Geometry check sheet. Reference: drawing and pictorial views, mm from the part's lowest x, y, z. A direction names the side the tool comes from. Round coordinates to 2 decimals unless told otherwise and drop trailing zeros. Write each loop counter-clockwise with the first axis right and the second up, starting at its lowest first coordinate (ties: lowest second). Pieces come first, ordered by that corner, then holes. Notation, with made-up numbers: (-11.5, 10.5) - (-4.5, 10.5) arc R34 cw to (-4.5, 46.5) - close; hole circle Ø5 at (2, -13.5). An arc over 180 degrees is marked (long way). Return JSON: item names as keys, results as strings.
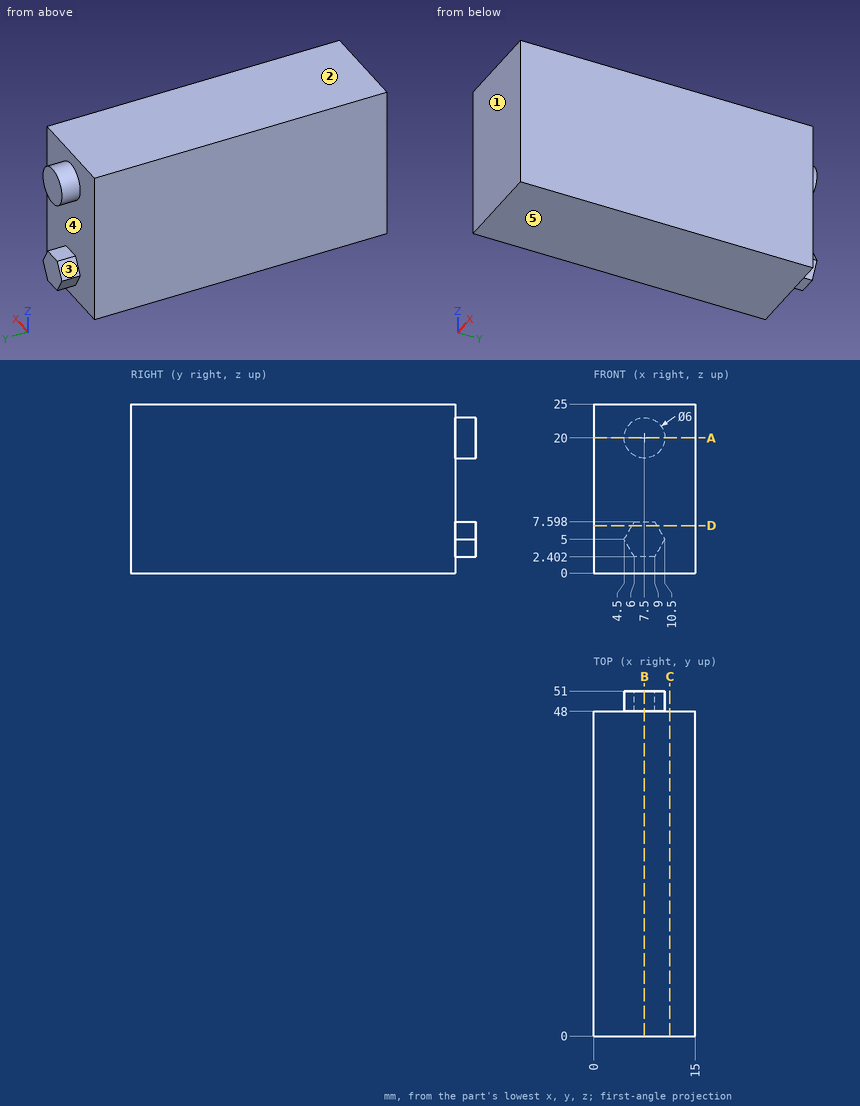
(1) Section check B-B, the plane x = 7.5. Enter the section's corners in (y, z), plus the area to 3 significant figures.
Response values:
{"outline": "(0, 0) - (48, 0) - (48, 2.4) - (51, 2.4) - (51, 7.6) - (48, 7.6) - (48, 17) - (51, 17) - (51, 23) - (48, 23) - (48, 25) - (0, 25) - close", "area": "1,230 mm^2"}
(2) Material ranges on line 1 along Y through (x, z) = (12.75, 12), recorded low to high. Write a range as [from, to].
Response values:
{"line 1": "y = [0, 48]"}
(3) Gauge pin test, flat ends, axial feed: pin 1 (1.5 mm diameter, centred on x = 8, y = 49.5, fed in from +Z); pin 2 (1.5 mm diameter, centred on x = 7.5, y = 49, fed in from -Z). Record the tip position at first contact, or that the pin passes through.
Response values:
{"pin 1": "stops at z = 23", "pin 2": "stops at z = 2.4"}
(4) Section check C-C, the plane x = 11.25. Enter the section's corners in (y, z).
Response values:
{"outline": "(0, 0) - (48, 0) - (48, 25) - (0, 25) - close"}
(5) Release check for a two-part mould opening along Z. For the marked faces 1, 2 and 3 record: pulls with the +Z half, pulls with the -Z half, needs draft (parallel to the pull), parting line crosses it, or undercut.
Response values:
{"face 1": "needs draft", "face 2": "pulls with the +Z half", "face 3": "undercut"}
(6) Section check A-A, the plane z = 20. Enter the section's corners in (x, y), plus the area to 3 significant figures.
Response values:
{"outline": "(0, 0) - (15, 0) - (15, 48) - (10.5, 48) - (10.5, 51) - (4.5, 51) - (4.5, 48) - (0, 48) - close", "area": "738 mm^2"}
(7) Access from +Z, -Z, +X, -X, +Y, -Y to the whole of each face (thin tool, end or side, straight path). Record for the marked faces 4 and 5.
Response values:
{"face 4": "+Y", "face 5": "-Z, +X, -X, +Y, -Y"}
(8) Section check D-D, the plane z = 7. Enter the section's corners in (x, y).
Response values:
{"outline": "(0, 0) - (15, 0) - (15, 48) - (9.35, 48) - (9.35, 51) - (5.65, 51) - (5.65, 48) - (0, 48) - close"}
